Geometry: see drawing. Coordinates: mm, zero at the bounding-box minimum. Give positions to 0.01 mm unless a question says otherwise; leave off trailing zeros. Write each loop counter-clockwise with the first axis right and the second up, starting at its lowest first coordinate (ties: lowest second). Pieces come first, ordered by that corner, then holes. Notation, with made-up numbers: M -20,6 L -11,6 A10 cw -11,13 Z; hole C 63,-11.5 d10. An arc over 180 degrees is marked long. Use a Markdown table: item, result. Add a question column.
1) Section B-B on z = 12.7. Return the cut outline in (x, y) (1 decimal), then the cut area to 3 significant figures.
2) Section C-C on y = 41.5. Return the cut outline in (x, z), then the cut area to 3 significant figures.
3) Pin query (flat end, axial travel): pin 1 (1.5 mm diameter, centred on x = 128, y = 1.5, fed in from -Z); pin 2 (2.5 mm diameter, centred on x = 33, y = 12.5, fed in from +Z); pin 3 (13 mm diameter, centred on x = 155, z = 195, fed in from +Y). Return the tip coordinate at first contact, or that it passes through.
4) Section D-D on y = 8. Return the cut outline in (x, z) (1 decimal), then the cut area to 3 significant figures.
5) Line query: line 1 (X direction, y = 1, z = 265); line 2 (X direction, y = 12.5, z = 251); line 3 (Y direction, x = 171.25, z = 260). Output: solid intervals per line, ascending.
6) Section A-A on x = 20. Return the cut outline in (y, z), then the cut area to 3 significant figures.
7) Draft query along X for the marked faces 1, 2, 3 and 4. Return one class per face: +X half, -X half, draft (parallel to the pull), parting line (faces both ways), or undercut.
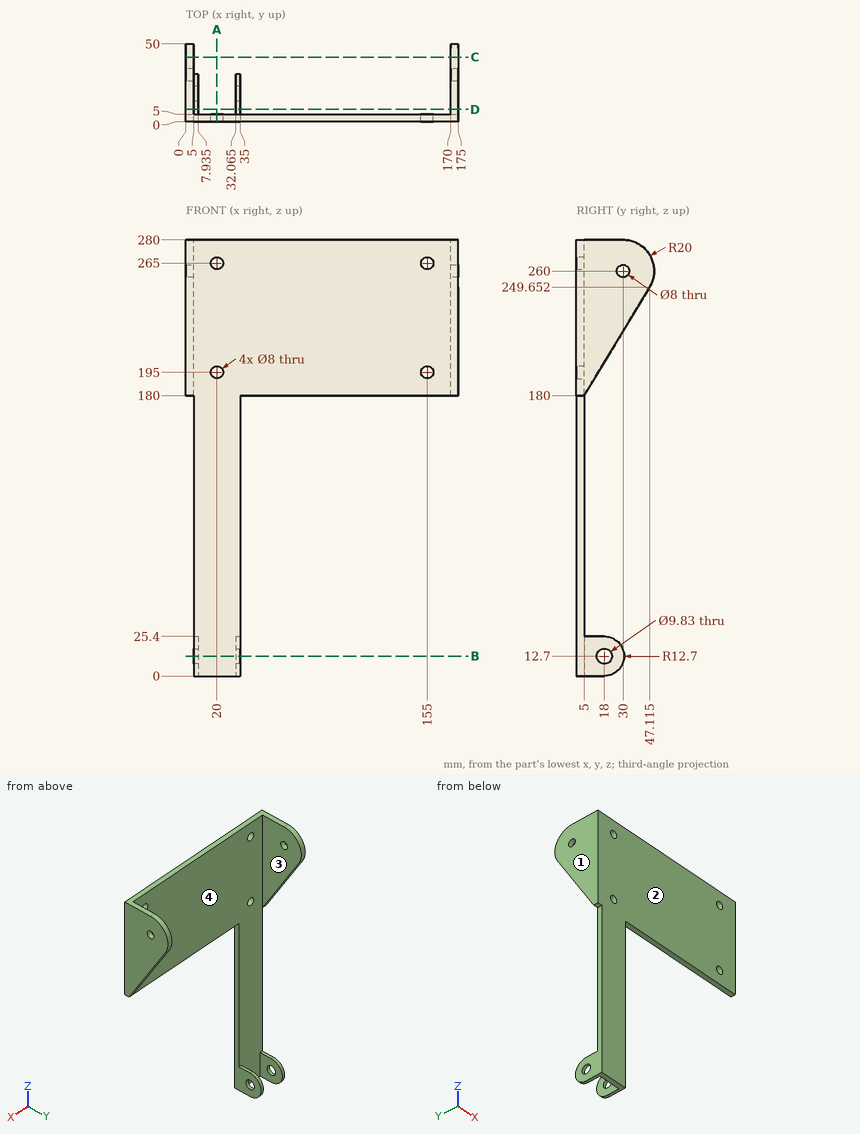
Found:
| question | item | result |
|---|---|---|
| 1 | outline | M 5,0 L 35,0 L 35,13.1 L 32.1,13.1 L 32.1,5 L 7.9,5 L 7.9,13.1 L 5,13.1 Z; M 5,22.9 L 7.9,22.9 L 7.9,30.7 L 5,30.7 Z; M 32.1,22.9 L 35,22.9 L 35,30.7 L 32.1,30.7 Z |
| 1 | area | 243 mm² |
| 2 | outline | M 0,240.37 L 5,240.37 L 5,276.36 L 0,276.36 Z; M 170,240.37 L 175,240.37 L 175,276.36 L 170,276.36 Z |
| 2 | area | 360 mm² |
| 3 | pin 1 | z = 180 |
| 3 | pin 2 | z = 25.4 |
| 3 | pin 3 | y = 5 |
| 4 | outline | M 0,185 L 5,185 L 5,280 L 0,280 Z; M 5,0 L 7.9,0 L 7.9,25.4 L 5,25.4 Z; M 32.1,0 L 35,0 L 35,25.4 L 32.1,25.4 Z; M 170,185 L 175,185 L 175,280 L 170,280 Z |
| 4 | area | 1,100 mm² |
| 5 | line 1 | 0 to 16, 24 to 151, 159 to 175 |
| 5 | line 2 | 0 to 5, 170 to 175 |
| 5 | line 3 | 0 to 26, 34 to 50 |
| 6 | outline | M 0,0 L 5,0 L 5,191 L 0,191 Z; M 0,199 L 5,199 L 5,261 L 0,261 Z; M 0,269 L 5,269 L 5,280 L 0,280 Z |
| 6 | area | 1,320 mm² |
| 7 | face 1 | -X half |
| 7 | face 2 | draft |
| 7 | face 3 | undercut |
| 7 | face 4 | undercut |
